Geometry: see drawing. Coordinates: mm, zero at the bounding-box minimum. Round coordinates to 2 decimals unless told otherwise and drop trailing zeros. Write each loop counter-clockwise with the first axis right and the second up, starting at its lowest first coordinate (ties: lowest second). Pieces come first, ordered by that corner, then holes. Notation, with made-up numbers: M -6,15 L -1,15 A12 ccw -1,37 Z; hole C -32.75,25 d5. An arc over 180 degrees is marked long. Use a Markdown table: item, result.
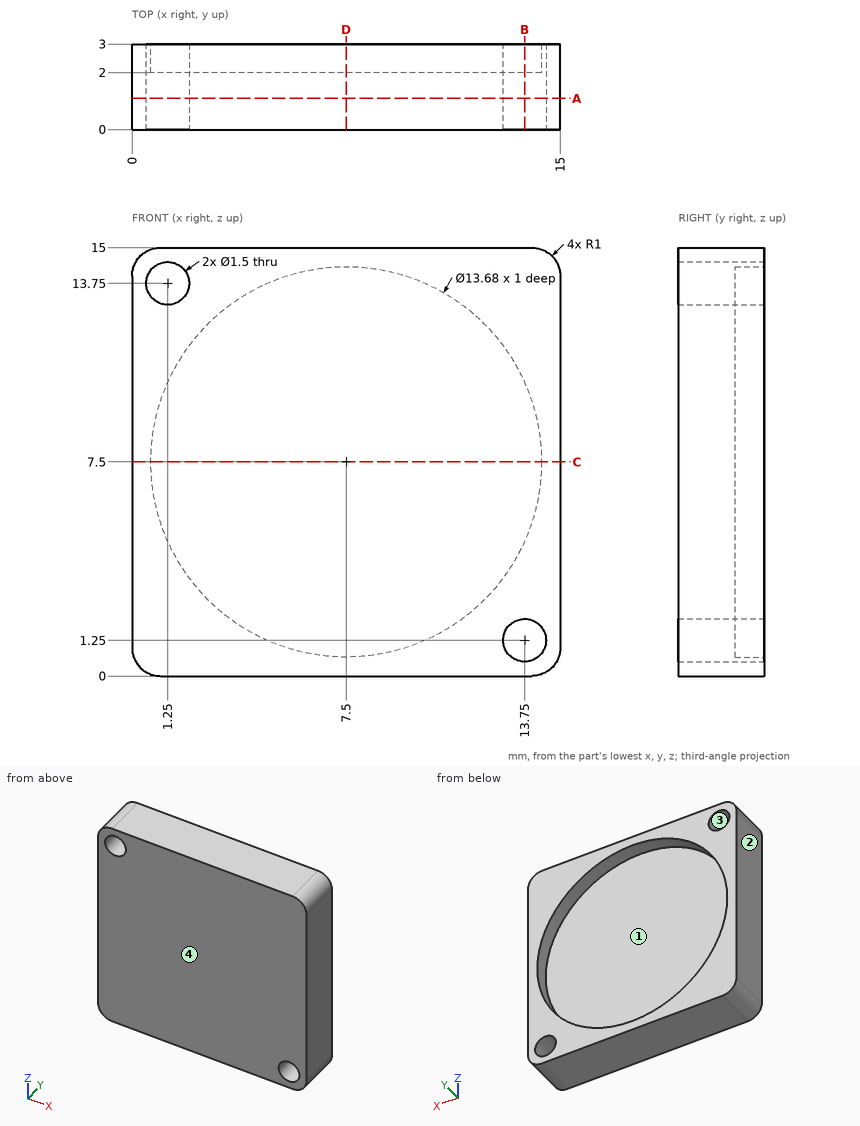
Q1. Section A-A on y = 1.1. Return loops of the section in (x, z), plus the area to 3 significant figures.
Results are:
| item | result |
|---|---|
| outline | M 0,1 A1 ccw 1,0 L 14,0 A1 ccw 15,1 L 15,14 A1 ccw 14,15 L 1,15 A1 ccw 0,14 Z; hole C 1.25,13.75 d1.5; hole C 13.75,1.25 d1.5 |
| area | 221 mm^2 |
Q2. Line query: L1, parallel to X at y = 1.45, z = 13.75; L2, parallel to Z at x = 7.5, y = 2.8; L3, parallel to Z at x = 13.75, y = 2.2. Output: solid intervals per line, ascending.
Results are:
| item | result |
|---|---|
| L1 | 0 to 0.5, 2 to 15 |
| L2 | 0 to 0.66, 14.34 to 15 |
| L3 | 0 to 0.5, 2 to 4.72, 10.28 to 15 |
Q3. Section C-C on z = 7.5. Return loops of the section in (x, y), plus the area to 3 significant figures.
Results are:
| item | result |
|---|---|
| outline | M 0,0 L 15,0 L 15,3 L 14.34,3 L 14.34,2 L 0.66,2 L 0.66,3 L 0,3 Z |
| area | 31.3 mm^2 |
Q4. Mould query, pull axis X, two halves, no side actions, for the marked faces 1, 2, 3 and 4. Classes: +X half, -X half, draft (parallel to the pull), parting line (faces both ways), or undercut.
Results are:
| item | result |
|---|---|
| face 1 | undercut |
| face 2 | -X half |
| face 3 | undercut |
| face 4 | draft |
Q5. First-contact query: pin 1 Ø4 at (x, z) = (4.5, 8) entering from +Y. Flat tip, straight axial feed; report the tip coordinate or a pass-through.
Results are:
| item | result |
|---|---|
| pin 1 | y = 2 |
Q6. Section D-D on x = 7.5. Return loops of the section in (y, z), plus the area to 3 significant figures.
Results are:
| item | result |
|---|---|
| outline | M 0,0 L 3,0 L 3,0.66 L 2,0.66 L 2,14.34 L 3,14.34 L 3,15 L 0,15 Z |
| area | 31.3 mm^2 |
Q7. Section B-B on x = 13.75. Return loops of the section in (y, z).
Results are:
| item | result |
|---|---|
| outline | M 0,0 L 3,0 L 3,0.5 L 0,0.5 Z; M 0,2 L 3,2 L 3,4.72 L 2,4.72 L 2,10.28 L 3,10.28 L 3,15 L 0,15 Z |
